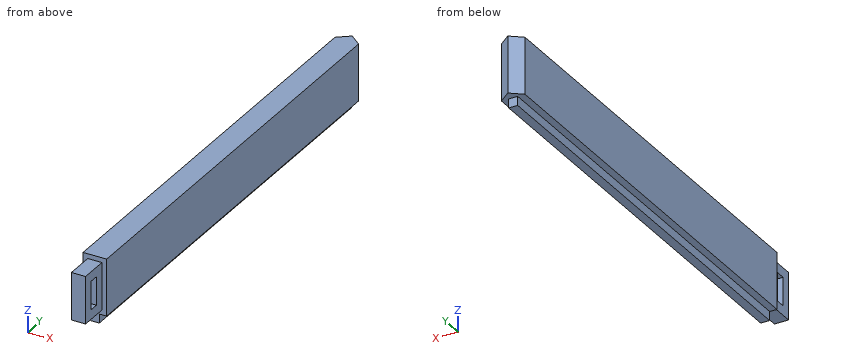
from build123d import *

# Parameters (mm, degrees)
SKETCH_1_W               = 5
SKETCH_1_H               = 92.4
EXTRUDE_1_DEPTH          = 12
EXTRUDE_2_DEPTH          = 1.9
SKETCH_3_W               = 3
SKETCH_3_H               = 2
SKETCH_3_H_2             = 6
EXTRUDE_3_DEPTH          = 6
CUT_EXTRUDE_1_DEPTH      = 100.209676947
CUT_EXTRUDE_1_DEPTH_BACK = 3
SKETCH_4_W               = 6
SKETCH_4_H               = 2


with BuildPart() as part:
    # Sketch 1 → Extrude 1 (new body)
    with BuildSketch(Plane.XY):
        with Locations((2.5, -46.2)):
            Rectangle(SKETCH_1_W, SKETCH_1_H)
        Polygon((0, 0), (2.5, 0), (2.5, 1.997498436), align=None)
        Polygon((2.5, 1.997498436), (2.5, 0), (5, 0), align=None)
    extrude(amount=EXTRUDE_1_DEPTH)

    # Sketch 2 → Extrude 2 (add)
    with BuildSketch(Plane(origin=(0, 0, 0), x_dir=(-1, 0, 0), z_dir=(0, 0, -1))):
        Polygon((-1.55, 0), (-3.45, 0), (-3.45, -1.400450224), (-3.45, -92.4), (-1.55, -92.4), (-1.55, -1.477736038), align=None)
    extrude(amount=EXTRUDE_2_DEPTH)

    # Sketch 3 → Extrude 3 (add)
    with BuildSketch(Plane.XZ.offset(92.4)):
        with Locations((2.5, 10)):
            Rectangle(SKETCH_3_W, SKETCH_3_H)
        with Locations((2.5, 6)):
            Rectangle(SKETCH_3_W, SKETCH_3_H_2)
        with Locations((2.5, 2)):
            Rectangle(SKETCH_3_W, SKETCH_3_H)
    extrude(amount=EXTRUDE_3_DEPTH)

    # Sketch 4 → Cut-Extrude 1 (cut, two sides: drawn at the far end of the back side and taken through both)
    with BuildSketch(Plane(origin=(4, 0, 0), x_dir=(0, 0, -1), z_dir=(1, 0, 0)).offset(-CUT_EXTRUDE_1_DEPTH_BACK)):
        with Locations((-6, -95.4)):
            Rectangle(SKETCH_4_W, SKETCH_4_H)
    extrude(amount=CUT_EXTRUDE_1_DEPTH + CUT_EXTRUDE_1_DEPTH_BACK, mode=Mode.SUBTRACT)


solid = part.part
Here's how the part is built. I have some questions about the finished solid (model axes, mm). Coordinates: 2 decimals unless noted, no trailing zeros. Write each loop counter-clockwise with the first axis right and the second up, starting at its lowest first coordinate (ties: lowest second). Pieces come first, ordered by that corner, then holes.
Item 1: I want a section at A-A on z = 6.5. Write out the boundary of the cut face in (x, y), and give its area (3 significant figures).
Item 2: I want a section at C-C on z = -1. Write out the boundary of the cut face in (x, y).
Item 3: I want a section at B-B on y = -88. Write out the boundary of the cut face in (x, z), and give its area (3 significant figures).
Item 4: If I drill on line 1 (Z direction, x = 3.8, y = -93); line 2 (Y direction, x = 2, z = -1); line 3 (Z direction, x = 4.1, y = -19.5), over which ranges is the centre line in solid material (lowest first)?
Item 5: Will these pins go through, and if not, where does the flat tip stop? pin 1 (2.5 mm diameter, centred on x = 3, z = 5, fed in from +Y); pin 2 (0.9 mm diameter, centred on x = 3, y = -94, fed in from +Z); pin 3 (3 mm diameter, centred on y = -94.5, z = 6.5, fed in from +X); pin 4 (3 mm diameter, centred on y = -41.5, z = 5, fed in from -X).
Findings below:
1. outline: (0, -92.4) - (1, -92.4) - (1, -94.4) - (4, -94.4) - (4, -92.4) - (5, -92.4) - (5, 0) - (2.5, 2) - (0, 0) - close; (1, -98.4) - (4, -98.4) - (4, -96.4) - (1, -96.4) - close
1. area: 479 mm2
2. outline: (1.55, -92.4) - (3.45, -92.4) - (3.45, 0) - (1.55, 0) - close
3. outline: (0, 0) - (1.55, 0) - (1.55, -1.9) - (3.45, -1.9) - (3.45, 0) - (5, 0) - (5, 12) - (0, 12) - close
3. area: 63.6 mm2
4. line 1: z = 1 to 11
4. line 2: y = -92.4 to 0
4. line 3: z = 0 to 12
5. pin 1: stops at y = 2
5. pin 2: stops at z = 11
5. pin 3: stops at x = 4
5. pin 4: stops at x = 0
